Work out the finished part from the listing and answer in its coordinate system (mm). Face numbers are marked on the shaded views. A direction names the side the tool comes from. Coordinates: 2 decimals unless noted, no trailing zeros. Loops run counter-clockwise (first coordinate to the right, second up) from the corner with the lowest first, then second, coordinate; pieces in that order, holes last. Notation, with made-up numbers: M -35,13 L -12,13 A18 cw -12,28 Z; hole C 70,78 d9. An arc over 180 degrees is marked long. Write each question's results on one line, items separated by ' | '.
Autodesk Inventor part; units mm, degrees
ref_plane "YZ Plane" through (0, 0, 0) normal (1, 0, 0) x (0, 1, 0)
ref_plane "XZ Plane" through (0, 0, 0) normal (0, 1, 0) x (-1, 0, 0)
ref_plane "XY Plane" through (0, 0, 0) normal (0, 0, 1) x (1, 0, 0)
sketch "Skizze1" plane through (0, 0, 0) normal (0, 0, 1) x (1, 0, 0)
  line L0 (-50.8, 26.67) -> (50.8, 26.67)
  line L1 (50.8, 26.67) -> (50.8, -26.67)
  line L2 (50.8, -26.67) -> (-50.8, -26.67)
  line L3 (-50.8, -26.67) -> (-50.8, 26.67)
  line L4 (0, -37.338) -> (0, 37.338)
  line L5 (-78.32, 0) -> (72.32, 0)
  circle A0 centre (-35.56, 24.13) radius 1.6
  circle A1 centre (-36.83, -24.13) radius 1.6
  circle A2 centre (39.37, 24.13) radius 1.6
  circle A3 centre (45.72, -24.13) radius 1.6
  circle A4 centre (15.24, -19.05) radius 1.6
  line L6 (-29.812, 25.1729) -> (-4.812, 25.1729)
  line L7 (-4.812, 25.1729) -> (-4.812, 22.67)
  line L8 (-4.812, 22.67) -> (-29.812, 22.67)
  line L9 (-29.812, 22.67) -> (-29.812, 25.1729)
  line L10 (-1.4087, 25.1729) -> (13.5913, 25.1729)
  line L11 (13.5913, 25.1729) -> (13.5913, 22.6729)
  line L12 (13.5913, 22.6729) -> (-1.4087, 22.6729)
  line L13 (-1.4087, 22.6729) -> (-1.4087, 25.1729)
  line L14 (16.84, 25.1729) -> (35.34, 25.1729)
  line L15 (35.34, 25.1729) -> (35.34, 22.6729)
  line L16 (35.34, 22.6729) -> (16.84, 22.6729)
  line L17 (16.84, 22.6729) -> (16.84, 25.1729)
  line L18 (46.87, 24.13) -> (43.37, 24.13)
  line L19 (43.37, 24.13) -> (43.37, -20.87)
  line L20 (43.37, -20.87) -> (46.87, -20.87)
  line L21 (46.87, -20.87) -> (46.87, 24.13)
  line L22 (40.4611, -25.17) -> (22.2148, -25.17)
  line L23 (22.2148, -25.17) -> (22.2148, -22.67)
  line L24 (22.2148, -22.67) -> (40.4611, -22.67)
  line L25 (40.4611, -22.67) -> (40.4611, -25.17)
  line L26 (19.229, -22.67) -> (1.6551, -22.67)
  line L27 (1.6551, -22.67) -> (1.6551, -25.17)
  line L28 (1.6551, -25.17) -> (19.229, -25.17)
  line L29 (19.229, -25.17) -> (19.229, -22.67)
  line L30 (-1.4087, -22.67) -> (-17.312, -22.67)
  line L31 (-17.312, -22.67) -> (-17.312, -25.17)
  line L32 (-17.312, -25.17) -> (-1.4087, -25.17)
  line L33 (-1.4087, -25.17) -> (-1.4087, -22.67)
  line L34 (-56.8, 17.67) -> (-40.8, 17.67)
  line L35 (-40.8, 17.67) -> (-40.8, 7.67)
  line L36 (-40.8, 7.67) -> (-56.8, 7.67)
  line L37 (-56.8, 7.67) -> (-56.8, 17.67)
  line L38 (-52.8, -14.67) -> (-38.8, -14.67)
  line L39 (-38.8, -14.67) -> (-38.8, -23.17)
  line L40 (-38.8, -23.17) -> (-52.8, -23.17)
  line L41 (-52.8, -23.17) -> (-52.8, -14.67)
  point P0 (0, 0)
  point P1 (-50.8, 17.67)
  point P2 (-50.8, 7.67)
  point P3 (-50.8, -14.67)
  point P4 (-50.8, -23.17)
  dimension "d0" = 101.6
  dimension "d1" = 53.34
  dimension "d2" = 3.2
  dimension "d3" = 15.24
  dimension "d4" = 3.2
  dimension "d5" = 13.97
  dimension "d6" = 2.54
  dimension "d7" = 48.26
  dimension "d8" = 3.2
  dimension "d9" = 90.17
  dimension "d10" = 3.2
  dimension "d11" = 96.52
  dimension "d12" = 3.2
  dimension "d13" = 66.04
  dimension "d14" = 7.62
  dimension "d15" = 25
  dimension "d16" = 4
  dimension "d17" = 15
  dimension "d18" = 2.5
  dimension "d19" = 18.5
  dimension "d20" = 3.5
  dimension "d21" = 45
  dimension "d22" = 4
  dimension "d23" = 2.5
  dimension "d24" = 4
  dimension "d25" = 9
  dimension "d26" = 10
  dimension "d27" = 16
  dimension "d28" = 6
  dimension "d29" = 8.5
  dimension "d30" = 3.5
  dimension "d31" = 14
  dimension "d32" = 2
extrude "Extrusion1" add sketch "Skizze1" along normal blind 1 contours L0 L4 L10 L13 L12 L5 L3 L36 L35 L34 | L0 L1 L5 L21 L18 L19 L4 L12 L11 L10 | L1 L2 L4 L5 L19 L20 L21 | L5 L4 L2 L3 L40 L39 L38
extrude "Extrusion2" add sketch "Skizze1" along normal blind 8 contours L10 L11 L12 L4 | L4 L12 L13 L10 | L6 L7 L8 L9 | L14 L15 L16 L17 | L22 L23 L24 L25 | L29 L28 L27 L26 | L33 L32 L31 L30
extrude "Extrusion3" add sketch "Skizze1" along normal blind 8 contours L21 L20 L19 L5 | L5 L19 L18 L21
extrude "Extrusion5" add sketch "Skizze1" along normal blind 10 contours L34 L35 L36 L3 | L3 L36 L37 L34
extrude "Extrusion6" add sketch "Skizze1" along normal blind 10 contours L38 L39 L40 L3 | L3 L40 L41 L38
properties part number "ArduinoMega"
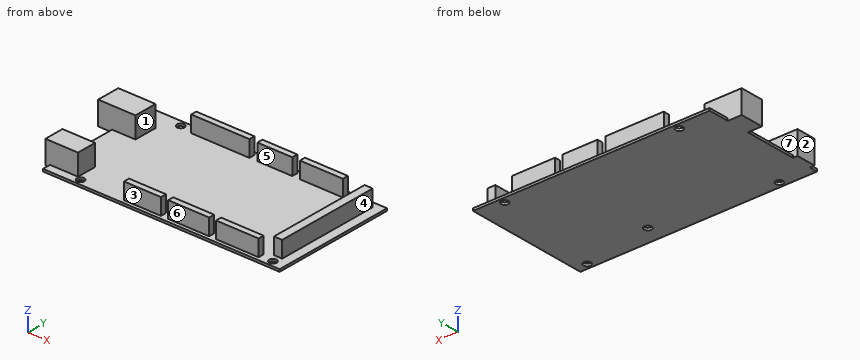
1) Find section B-B, the plane x = 39.37. Give the vertices of the cut face in (y, z), and give its area (3 significant figures).
Check result:
outline: M -26.67,0 L 22.53,0 L 22.53,1 L -22.67,1 L -22.67,8 L -25.17,8 L -25.17,1 L -26.67,1 Z; M 25.73,0 L 26.67,0 L 26.67,1 L 25.73,1 Z | area: 67.6 mm^2
2) For a pull along Y with two mould halves and no side action, classify the marked faces 4, 5, 6 and 7 as released by +Y, released by -Y, zero draft, split by the parting line, or undercut.
Check result:
face 4: zero draft | face 5: undercut | face 6: released by -Y | face 7: undercut
3) Find section C-C, the plane y = -19.05. Give the vertices of the cut face in (x, z).
Check result:
outline: M -52.8,0 L 13.64,0 L 13.64,1 L -38.8,1 L -38.8,10 L -52.8,10 Z; M 16.84,0 L 50.8,0 L 50.8,1 L 46.87,1 L 46.87,8 L 43.37,8 L 43.37,1 L 16.84,1 Z
4) Straight lines are drawn through the part: probe 1 along X at (y, z) = (23, 7.5); probe 2 along Y at (x, z) = (15.24, 0.25); probe 3 along Y at (x, z) = (35, 2.5). For each, find the intervals that lie inside material, in ascending order. Write a range as [from, to].
Check result:
probe 1: [-29.81, -4.81], [-1.41, 13.59], [16.84, 35.34], [43.37, 46.87] | probe 2: [-26.67, -20.65], [-17.45, 26.67] | probe 3: [-25.17, -22.67], [22.67, 25.17]
5) Find section D-D, the plane y = 4.5. Give the vertices of the cut face in (x, z).
Check result:
outline: M -50.8,0 L 50.8,0 L 50.8,1 L 46.87,1 L 46.87,8 L 43.37,8 L 43.37,1 L -50.8,1 Z
6) Which of the six approach directions +Z, -Z, +X, -X, +Y, -Y give full straight-line access (tool end or side, diameter ignored) to the marked faces 1, 2 and 3?
Check result:
face 1: +Z, +Y | face 2: +Z, -Z, -X, -Y | face 3: +Z, +X, -X, -Y
7) Given pin 1 Ø6 at (y, z) = (-3.5, 7.5) entering from +X; pin 2 Ø3.5 at (x, z) = (-8.5, 3.5) entering from -Y; pin 3 Ø3 at (x, y) = (6, -16.5) entering from -Z; pin 4 Ø0.8 at (x, y) = (24, 24) entering from +Z, each flat-ended and moving along its own axis, determine where each tip first touches the part or whether it passes through.
Check result:
pin 1: x = 46.87 | pin 2: y = -25.17 | pin 3: z = 0 | pin 4: z = 8
8) Find section A-A, the plane z = 9. Give the vertices of the cut face in (x, y).
Check result:
outline: M -56.8,7.67 L -40.8,7.67 L -40.8,17.67 L -56.8,17.67 Z; M -52.8,-23.17 L -38.8,-23.17 L -38.8,-14.67 L -52.8,-14.67 Z
